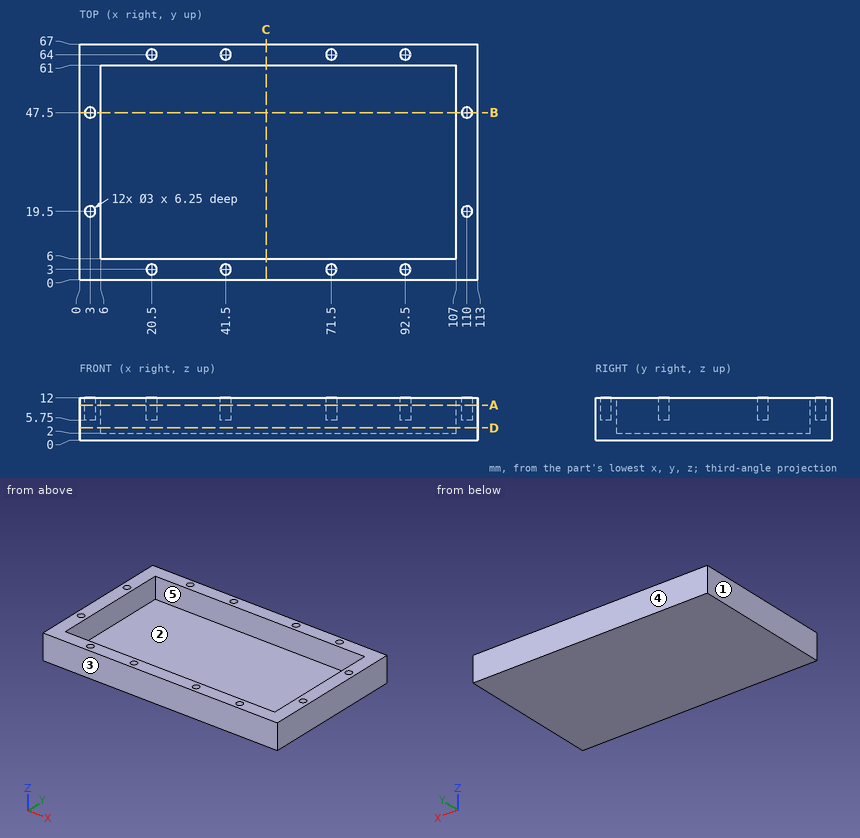
Design review of the part shown in the three views and the two pictorial views. Dimensions are in mm from the part's minimum x, y and z. A direction names the side the tool comes from. Coordinates: 2 decimals unless noted, no trailing zeros. Write each loop counter-clockwise with the first axis right and the second up, starting at its lowest first coordinate (ties: lowest second). Pieces come first, ordered by that corner, then holes.
1) We need section B-B on y = 47.5. State the section outline as (x, z) points.
2) Machinability: for the marked faces 4 and 5, which of the approach directions +Z, -Z, +X, -X, +Y, -Y give a long, thin tool a straight path to every point of the face, cutting with its end or side? Answer none if there is none.
3) Clearance check with flat-ended pins moving along their axes: pin 1 Ø4 at (x, y) = (49, 42) entering from +Z; pin 2 Ø1.8 at (x, y) = (92.5, 3) entering from +Z. State where each tip first meets the part, or that it passes through.
4) We need section D-D on z = 3.5. State the section outline as (x, y) points, then the cut area to 3 significant figures.
5) We need section C-C on x = 53. State the section outline as (y, z) points, then the cut area to 3 significant figures.
6) The part is to be moulded in two halves that separate along Y. For the marked faces 1, 2 and 3, say which applies: pulls with the +Y half, pulls with the -Y half, needs draft (parallel to the pull), parting line crosses it, or undercut.
7) We need section A-A on z = 10. Count the separate pieces of the cut face and the enclosed holes in it, then the cut area to 3 significant figures.
8) To check wall thickness, follow probe 1 along Y at (x, z) = (20.5, 7); probe 2 along X at (y, z) = (64, 9.75); probe 3 along Y at (x, z) = (73, 3.5). State the ranges of each line that lie inside material, in increasing order.
Answer list:
1. outline: (0, 0) - (113, 0) - (113, 12) - (111.5, 12) - (111.5, 5.75) - (108.5, 5.75) - (108.5, 12) - (107, 12) - (107, 2) - (6, 2) - (6, 12) - (4.5, 12) - (4.5, 5.75) - (1.5, 5.75) - (1.5, 12) - (0, 12) - close
2. face 4: +Z, -Z, +X, -X, +Y
2. face 5: +Z
3. pin 1: stops at z = 2
3. pin 2: stops at z = 5.75
4. outline: (0, 0) - (113, 0) - (113, 67) - (0, 67) - close; hole (6, 6) - (107, 6) - (107, 61) - (6, 61) - close
4. area: 2,020 mm2
5. outline: (0, 0) - (67, 0) - (67, 12) - (61, 12) - (61, 2) - (6, 2) - (6, 12) - (0, 12) - close
5. area: 254 mm2
6. face 1: needs draft
6. face 2: undercut
6. face 3: pulls with the -Y half
7. separate pieces: 1
7. enclosed holes: 13
7. area: 1,930 mm2
8. probe 1: y = 0 to 1.5, 4.5 to 6, 61 to 62.5, 65.5 to 67
8. probe 2: x = 0 to 19, 22 to 40, 43 to 70, 73 to 91, 94 to 113
8. probe 3: y = 0 to 6, 61 to 67
